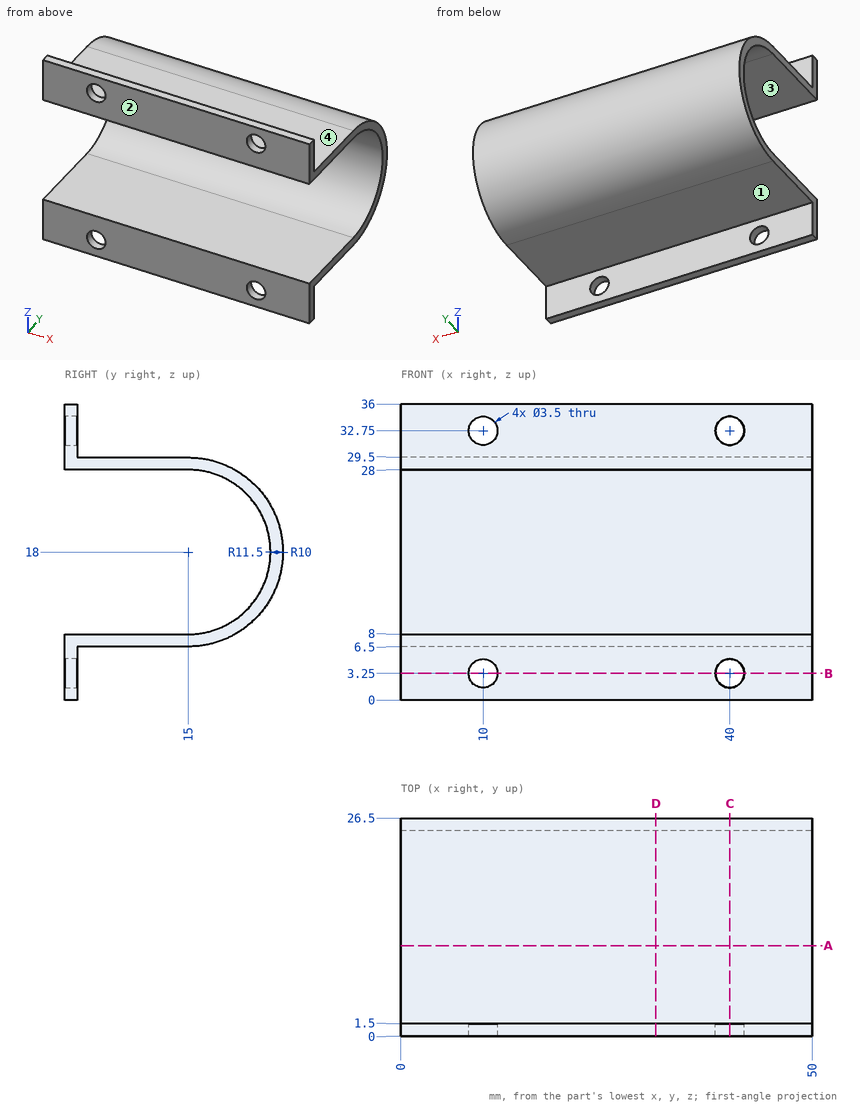
Study the drawing (mm; zero at the part's minimum x, y, z) and answer. A direction names the side the tool comes from. Coordinates: 2 decimals unless noted, no trailing zeros. Write each loop counter-clockwise with the first axis right and the second up, starting at its lowest first coordinate (ties: lowest second). Pieces come first, ordered by that corner, then holes. Notation, with made-up numbers: (0, 28) - (18, 28) arc R11 ccw to (18, 39) - close; hole circle Ø2 at (56.5, 88). An arc over 180 degrees is marked (long way). Answer as a JSON object with one key per item and string values.
Q1. Consider L1, parallel to X at y = 0.5, z = 32.75; L2, parallel to Z at x = 40, y = 0.5; L3, parallel to Z at x = 30.5, y = 12.5. Determine where each line is inside the solid, lowest interval first. Write a range as from..to.
Results list:
{"L1": "x = 0..8.25, 11.75..38.25, 41.75..50", "L2": "z = 0..1.5, 5..8, 28..31, 34.5..36", "L3": "z = 6.5..8, 28..29.5"}
Q2. Find section D-D (x = 31). Write down the section's boundary in (y, z).
Results list:
{"outline": "(0, 0) - (1.5, 0) - (1.5, 6.5) - (15, 6.5) arc R11.5 ccw to (15, 29.5) - (1.5, 29.5) - (1.5, 36) - (0, 36) - (0, 28) - (15, 28) arc R10 cw to (15, 8) - (0, 8) - close"}
Q3. Find section B-B (z = 3.25). Write down the section's boundary in (x, y).
Results list:
{"outline": "(0, 0) - (8.25, 0) - (8.25, 1.5) - (0, 1.5) - close; (11.75, 0) - (38.25, 0) - (38.25, 1.5) - (11.75, 1.5) - close; (41.75, 0) - (50, 0) - (50, 1.5) - (41.75, 1.5) - close"}
Q4. Given pin 1 Ø3 at (y, z) = (3.5, 9) entering from -X; pin 2 Ø3 at (x, z) = (22, 4) entering from +Y; pin 3 Ø1.5 at (x, y) = (21, 22.5) entering from -Z; pin 4 Ø12 at (x, y) = (26.5, 10) entering from +Z, each flat-ended and moving along its own axis, determine where each tip first touches the part or whether it passes through.
Results list:
{"pin 1": "stops at x = 0", "pin 2": "stops at y = 1.5", "pin 3": "stops at z = 8.69", "pin 4": "stops at z = 29.5"}
Q5. Which of the six approach directions +Z, -Z, +X, -X, +Y, -Y give full straight-line access (tool end or side, diameter ignored) to the marked faces 1, 2, 3 and 4?
Results list:
{"face 1": "-Z, +X, -X, +Y", "face 2": "+Z, -Z, +X, -X, -Y", "face 3": "+X, -X, -Y", "face 4": "+Z, +X, -X, +Y"}
Q6. Find section A-A (y = 11). Write down the section's boundary in (x, z), plus the area to 3 significant figures.
Results list:
{"outline": "(0, 6.5) - (50, 6.5) - (50, 8) - (0, 8) - close; (0, 28) - (50, 28) - (50, 29.5) - (0, 29.5) - close", "area": "150 mm^2"}
Q7. Find section C-C (x = 40). Write down the section's boundary in (y, z), plus the area to 3 significant figures.
Results list:
{"outline": "(0, 0) - (1.5, 0) - (1.5, 1.5) - (0, 1.5) - close; (0, 5) - (1.5, 5) - (1.5, 6.5) - (15, 6.5) arc R11.5 ccw to (15, 29.5) - (1.5, 29.5) - (1.5, 31) - (0, 31) - (0, 28) - (15, 28) arc R10 cw to (15, 8) - (0, 8) - close; (0, 34.5) - (1.5, 34.5) - (1.5, 36) - (0, 36) - close", "area": "105 mm^2"}
